```python
from build123d import *

# Parameters (mm, degrees)
SKETCH_W     = 76
SKETCH_H     = 76
SKETCH_W_2   = 74
SKETCH_H_2   = 74
PAD_DEPTH    = 15
PAD001_DEPTH = 15
PAD002_DEPTH = 76
PAD004_DEPTH = 76


with BuildPart() as part:
    # Sketch → Pad (new body)
    with BuildSketch(Plane.XY):
        Rectangle(SKETCH_W, SKETCH_H)
        Rectangle(SKETCH_W_2, SKETCH_H_2, mode=Mode.SUBTRACT)
    extrude(amount=PAD_DEPTH)

    # Sketch001 → Pad001 (join)
    with BuildSketch(Plane.XY):
        Polygon((-17.5, 37), (-17.5, 12.333333), (-17.5, -37), (-19.5, -37), (-19.5, 12.333333), (-19.5, 37), align=None)
        Polygon((-37, 19.5), (-12.333333, 19.5), (37, 19.5), (37, 17.5), (-12.333333, 17.5), (-37, 17.5), align=None)
        Polygon((19.5, 37), (19.5, 12.333333), (19.5, -37), (17.5, -37), (17.5, 12.333333), (17.5, 37), align=None)
        Polygon((-37, -17.5), (-12.333333, -17.5), (37, -17.5), (37, -19.5), (-12.333333, -19.5), (-37, -19.5), align=None)
        Polygon((-1, -37), (-1, -12.333333), (-1, 37), (1, 37), (1, -12.333333), (1, -37), align=None)
        Polygon((-37, 1), (-12.333333, 1), (37, 1), (37, -1), (-12.333333, -1), (-37, -1), align=None)
    extrude(amount=PAD001_DEPTH)

    # Sketch002 (on Face1 of Pad001) → Pad002 (join)
    with BuildSketch(Plane.XZ.offset(38)):
        Polygon((-39, 8), (-38, 8), (-38, 7), (-39, 7), (-39, 5.5), (-38, 5.5), (-38, 0), (-37, 0), (-37, 15), (-38, 15), align=None)
        Polygon((38, 8.000002), (39, 8.000002), (38, 15.000002), (37, 15), (37, 0), (38, 0), (38, 5.500002), (39, 5.500002), (39, 7.000002), (38, 7.000002), align=None)
    extrude(amount=-PAD002_DEPTH)

    # Sketch004 (on Face4 of Pad) → Pad004 (join)
    with BuildSketch(Plane(origin=(-38, 0, 0), x_dir=(0, -1, 0), z_dir=(-1, 0, 0))):
        Polygon((38, 15), (37, 15), (37, 8), (39, 8), align=None)
    extrude(amount=-PAD004_DEPTH)


solid = part.part
```
Could you check a few things on this model? Use its own coordinates, in mm. Round coordinates to 2 decimals unless told otherwise and drop trailing zeros. Loops run counter-clockwise (first coordinate to the right, second up) from the corner with the lowest first, then second, coordinate; pieces in that order, holes last. Notation, with made-up numbers: (60, 68.25) - (103, 68.25) arc R33 cw to (103, 99.25) - close; hole circle Ø3 at (-40, -34). An arc over 180 degrees is marked (long way). Answer in a Markdown table with one row per item. Add a question column.
(1) If we section it at B-B (x = 20.5): Please give me the cut outline in (y, z).
(2) I'm going to push flat-ended pins straight in: pin 1 (3 mm diameter, centred on y = 4, z = 1.5, fed in from +X); pin 2 (0.8 mm diameter, centred on x = -38.5, y = 5, fed in from -Z); pin 3 (3 mm diameter, centred on y = 13.5, z = 2.5, fed in from -X); pin 4 (4 mm diameter, centred on x = 8.5, y = 14.5, fed in from -Z). Where does each tip first touch, or does it pass through?
(3) I need wall thicknesses on line 1 along Y through (x, z) = (29, 7); line 2 along X through (y, z) = (-14.5, 10.5). Which ranges of each line are inside material? Lowest first, please.
(4) If we mould it in two halves opening along Y, with no side actions, what happens to faces 1 (the face through (-38.5, -0.5, 11.5)), 2 (the face through (-9, 17.5, 7))? For each: pulls with the +Y half, pulls with the -Y half, needs draft (parallel to the pull), parting line crosses it, or undercut.
(5) If we section it at A-A (y = 2.5): State how many separate pieces and enclosed holes the cut face has, plus the area to 3 significant figures.
Model answer:
| question | item | result |
|---|---|---|
| 1 | outline | (-39, 8) - (-38, 8) - (-38, 0) - (-37, 0) - (-37, 15) - (-38, 15) - close; (-19.5, 0) - (-17.5, 0) - (-17.5, 15) - (-19.5, 15) - close; (-1, 0) - (1, 0) - (1, 15) - (-1, 15) - close; (17.5, 0) - (19.5, 0) - (19.5, 15) - (17.5, 15) - close; (37, 0) - (38, 0) - (38, 15) - (37, 15) - close |
| 2 | pin 1 | stops at x = 38 |
| 2 | pin 2 | stops at z = 5.5 |
| 2 | pin 3 | stops at x = -38 |
| 2 | pin 4 | passes through |
| 3 | line 1 | y = -38 to -37, -19.5 to -17.5, -1 to 1, 17.5 to 19.5, 37 to 38 |
| 3 | line 2 | x = -38.64 to -37, -19.5 to -17.5, -1 to 1, 17.5 to 19.5, 37 to 38.64 |
| 4 | face 1 | needs draft |
| 4 | face 2 | undercut |
| 5 | separate pieces | 5 |
| 5 | enclosed holes | 0 |
| 5 | area | 130 mm² |
